from build123d import *

# Parameters (mm, degrees)
F0_R        = 5.25
F0_R_2      = 4.75
F1_DEPTH    = 16.5
F2_R        = 11.15
F2_R_2      = 11.7991480977
F3_DEPTH    = 7
F4_R        = 15
F5_R        = 15
F6_T1_DEPTH = 176.0234639037


# Not quite as in the source:
# - a fillet or chamfer that OpenCascade refuses, or shapes differently, is made with other operations: its cross-section is extruded or revolved along the edge and cut away or added


with BuildPart() as f1:
    # F0 (on Front) → F1 (new body)
    with BuildSketch(Plane.XZ):
        with BuildLine():
            Line((28.7001559958, 61.0160396297), (-111.2998440042, 61.0160396297))
            Line((-111.2998440042, 61.0160396297), (-111.2998440042, 14.5160396297))
            Line((-111.2998440042, 14.5160396297), (28.7001559958, 14.5160396297))
            Line((28.7001559958, 14.5160396297), (52.362193456, 43.3288254373))
            ThreePointArc((52.362193456, 43.3288254373), (53.9004778512, 54.793039046), (44.1501559958, 61.0160396297))
            Line((44.1501559958, 61.0160396297), (28.7001559958, 61.0160396297))
        make_face()
        with Locations((-95.1498440042, 30.3660396297)):
            Circle(F0_R, mode=Mode.SUBTRACT)
        with Locations((16.5501559958, 31.1660396297)):
            Circle(F0_R, mode=Mode.SUBTRACT)
        with Locations((-62.0498440042, 45.8660396297)):
            Circle(F0_R, mode=Mode.SUBTRACT)
        with Locations((-89.5498440042, 50.2660396297)):
            Circle(F0_R_2, mode=Mode.SUBTRACT)
        with Locations((-22.7498440042, 45.8660396297)):
            Circle(F0_R, mode=Mode.SUBTRACT)
        with Locations((44.1501559958, 50.2660396297)):
            Circle(F0_R_2, mode=Mode.SUBTRACT)
    extrude(amount=F1_DEPTH)

    # F2 (on face) → F3 (cut)
    with BuildSketch(Plane.XZ.offset(16.5)):
        with Locations((-95.1498440042, 30.3660396297)):
            Circle(F2_R)
        with Locations((-62.0498440042, 45.8660396297)):
            Circle(F2_R)
        with Locations((-22.7498440042, 45.8660396297)):
            Circle(F2_R_2)
        with Locations((16.5501559958, 31.1660396297)):
            Circle(F2_R_2)
    extrude(amount=-F3_DEPTH, mode=Mode.SUBTRACT)

    # F4
    f4_edges = [f1.edges().sort_by_distance(p)[0] for p in [
        (28.700156, -8.25, 14.51604),
    ]]
    fillet(f4_edges, radius=F4_R)

    # F5
    f5_edges = [f1.edges().sort_by_distance(p)[0] for p in [
        (-111.299844, -8.25, 14.51604),
    ]]
    fillet(f5_edges, radius=F5_R)

    # F6: chamfer of 4 on 1 edges, made by hand

    # F6_s2 → F6_t1 (cut)
    with BuildSketch(Plane.YZ.offset(-121.5865759561)):
        Polygon((0, 57.0160396297), (-4, 61.0160396297), (0, 61.0160396297), align=None)
    extrude(amount=F6_T1_DEPTH, mode=Mode.SUBTRACT)


solid = f1.part
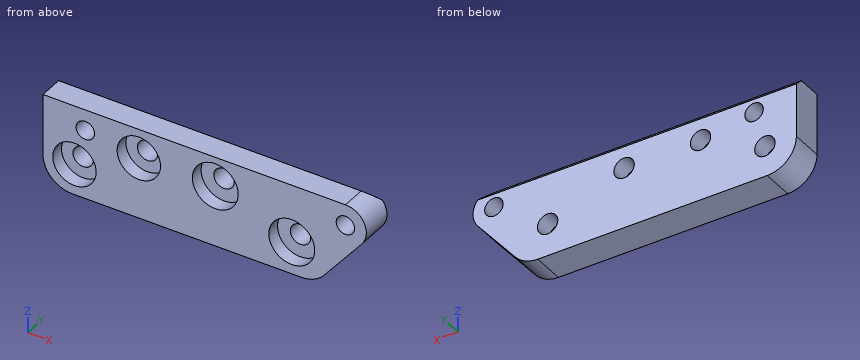
Source: CAD feature listing. Evaluate the final solid. Frame: model axes, mm. Round coordinates to 2 decimals unless told otherwise and drop trailing zeros. Loops run counter-clockwise (first coordinate to the right, second up) from the corner with the lowest first, then second, coordinate; pieces in that order, holes last.
Q1. Ray query, line 1 (X direction, y = -2, z = 48); line 2 (X direction, y = -8, z = 50); line 3 (X direction, y = -12.75, z = 32). Return the intervals inside material, ascending.
Q2. Section B-B, the plane y = -2. Return loops of the section in (x, z), plus the area to 3 significant figures.
Q3. First-contact query: P1, Ø12, axis at x = 22, z = 33, coming from the -Y side; P2, Ø19, axis at x = -25.5, z = 44.5, coming from the -Y side; P3, Ø1, axis at y = -10, z = 49, coming from the +X side; P4, Ø1.5, axis at y = -14.5, z = 25.5, coming from the -X side. Flat tips, straight axial feed; report the tip coordinate or a pass-through.
Q4. Section D-D, the plane y = -12. Return loops of the section in (x, z).
Q5. Section C-C, the plane z = 23. Return loops of the section in (x, y), plus the area to 3 significant figures.
Q6. Section A-A, the plane x = 41. Return loops of the section in (y, z).
Solutions:
1. line 1: x = -111.3 to -93.72, -85.38 to -66.85, -57.25 to -27.55, -17.95 to 39.98, 48.32 to 54.66
1. line 2: x = -111.3 to -94.29, -84.81 to -65.29, -58.81 to -25.99, -19.51 to 39.41, 48.89 to 54.9
1. line 3: x = -111.3 to -106.18, -84.12 to 4.78, 28.32 to 43.06
2. outline: (-111.3, 29.52) arc R15 ccw to (-96.3, 14.52) - (21.61, 14.52) arc R15 ccw to (33.2, 20) - (52.36, 43.33) arc R10.75 ccw to (50.4, 59.02) - (-111.3, 59.02) - close; hole circle Ø10.5 at (-95.15, 30.37); hole circle Ø9.5 at (-89.55, 50.27); hole circle Ø10.5 at (-62.05, 45.87); hole circle Ø10.5 at (-22.75, 45.87); hole circle Ø10.5 at (16.55, 31.17); hole circle Ø9.5 at (44.15, 50.27)
2. area: 6,420 mm2
3. P1: stops at y = -9.5
3. P2: stops at y = -16.5
3. P3: stops at x = 54.87
3. P4: stops at x = -110.94
4. outline: (-111.3, 29.52) arc R15 ccw to (-96.3, 14.52) - (21.61, 14.52) arc R15 ccw to (33.2, 20) - (52.36, 43.33) arc R10.75 ccw to (44.15, 61.02) - (-111.3, 61.02) - close; hole circle Ø22.3 at (-95.15, 30.37); hole circle Ø9.5 at (-89.55, 50.27); hole circle Ø22.3 at (-62.05, 45.87); hole circle Ø23.6 at (-22.75, 45.87); hole circle Ø23.6 at (16.55, 31.17); hole circle Ø9.5 at (44.15, 50.27)
5. outline: (-109.81, -16.5) - (-103.52, -16.5) - (-103.52, -9.5) - (-86.78, -9.5) - (-86.78, -16.5) - (8.03, -16.5) - (8.03, -9.5) - (25.07, -9.5) - (25.07, -16.5) - (35.67, -16.5) - (35.67, 0) - (-109.81, 0) - close
5. area: 2,160 mm2
6. outline: (-16.5, 29.49) - (0, 29.49) - (0, 46.71) - (-16.5, 46.71) - close; (-16.5, 53.82) - (0, 53.82) - (0, 57.02) - (-4, 61.02) - (-16.5, 61.02) - close
